The model under review builds one solid part; all positions refer to its coordinate system, in mm. Give positions to 0.01 mm unless a question says otherwise; leave off trailing zeros. Loops run counter-clockwise (first coordinate to the right, second up) from the corner with the lowest first, then second, coordinate; pieces in that order, holes last. Notation, with made-up numbers: (-11.5, 35) - (11.5, 35) arc R25 ccw to (11.5, 62) - close; hole circle Ø10 at (-10.5, -37). An arc over 180 degrees is marked (long way). Answer as a JSON object with one key per item and string values.
Autodesk Inventor part; units mm, degrees
ref_plane "YZ Plane" through (0, 0, 0) normal (1, 0, 0) x (0, 1, 0)
ref_plane "XZ Plane" through (0, 0, 0) normal (0, 1, 0) x (-1, 0, 0)
ref_plane "XY Plane" through (0, 0, 0) normal (0, 0, 1) x (1, 0, 0)
sketch "Sketch1" plane through (0, 0, 0) normal (0, 0, 1) x (1, 0, 0)
  line L0 (38.8522, 283.8417) -> (93.8522, 283.8417)
  line L1 (38.8522, 319.8417) -> (93.8522, 319.8417)
  arc A0 (10.8096, 312.4813) -> (10.8096, 291.2021) centre (13.6022, 301.8417) ccw
  line L2 (38.8522, 319.8417) -> (10.8096, 312.4813)
  line L3 (38.8522, 283.8417) -> (10.8096, 291.2021)
  arc A1 (121.8948, 291.2021) -> (121.8948, 312.4813) centre (119.1022, 301.8417) ccw
  line L4 (93.8522, 319.8417) -> (121.8948, 312.4813)
  line L5 (93.8522, 283.8417) -> (121.8948, 291.2021)
  circle A2 centre (13.6022, 301.8417) radius 5
  circle A3 centre (119.1022, 301.8417) radius 5
  circle A4 centre (58.3522, 316.3417) radius 1.5
  circle A5 centre (74.3522, 316.3417) radius 1.5
  circle A6 centre (58.3522, 287.3417) radius 1.5
  circle A7 centre (74.3522, 287.3417) radius 1.5
  dimension "d5" = 36
  dimension "d6" = 105.5
  dimension "d7" = 105.5
  dimension "d8" = 25.25
  dimension "d9" = 25.25
  dimension "d10" = 25.25
  dimension "d11" = 16
  dimension "d12" = 16
  dimension "d13" = 19.5
  dimension "d14" = 19.5
extrude "Extrusion1" add sketch "Sketch1" along normal blind 2.5
sketch "Sketch2" plane through (0, 0, 2.5) normal (0, 0, 1) x (1, 0, 0)
  circle A0 centre (13.6022, 301.8417) radius 5
  circle A1 centre (22.1022, 301.8417) radius 1
  point P0 (0, 0)
  dimension "d15" = 2
  dimension "d16" = 8.5
extrude "Extrusion2" cut sketch "Sketch2" against normal through all contours A1
pattern_circular "Circular Pattern1" count 8 over 360 about axis through (13.6022, 301.8417, 0) along (0, 0, 1) of "Extrusion2"
sketch "Sketch3" plane through (0, 0, 2.5) normal (0, 0, 1) x (1, 0, 0)
  circle A0 centre (5.1022, 301.8417) radius 1
  line L0 (93.8522, 319.8417) -> (38.8522, 319.8417)
  line L1 (66.3522, 319.8417) -> (66.3522, 283.8417)
  line L2 (38.8522, 283.8417) -> (93.8522, 283.8417)
  circle A1 centre (127.6022, 301.8417) radius 1
  point P0 (0, 0)
extrude "Extrusion3" cut sketch "Sketch3" against normal through all contours A1
pattern_circular "Circular Pattern2" count 8 over 360 about axis through (119.1022, 301.8417, 0) along (0, 0, 1) of "Extrusion3"
properties part number "Thigh" material "Aluminum-6061"
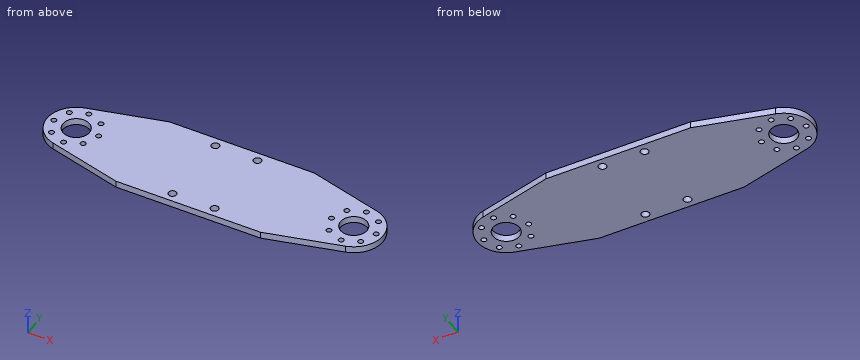
Q1. Consider section A-A, the plane y = 305.5. State the section outline as (x, z) points, plus the area to 3 significant figures.
Results:
{"outline": "(3.23, 0) - (10.19, 0) - (10.19, 2.5) - (3.23, 2.5) - close; (17.01, 0) - (115.69, 0) - (115.69, 2.5) - (17.01, 2.5) - close; (122.51, 0) - (129.48, 0) - (129.48, 2.5) - (122.51, 2.5) - close", "area": "282 mm^2"}
Q2. Consider section C-C, the plane y = 290. State the section outline as (x, z) points.
Results:
{"outline": "(15.39, 0) - (117.31, 0) - (117.31, 2.5) - (15.39, 2.5) - close"}
Q3. To check wall thickness, follow probe 1 along X at (y, z) = (303, 2.1); probe 2 along Y at (x, z) = (57.5, 2.25); probe 3 along X at (y, z) = (300, 1.1). State the ranges of each line that lie inside material, in increasing order. Write a range as [from, to].
Results:
{"probe 1": "x = [2.66, 8.74], [18.47, 114.24], [123.97, 130.04]", "probe 2": "y = [283.84, 286.11], [288.58, 315.11], [317.58, 319.84]", "probe 3": "x = [2.76, 8.95], [18.25, 114.45], [123.75, 129.95]"}
Q4. Consider section B-B, the plane z = 0.9. State how many separate pieces and enclosed holes the cut face has, plus the area to 3 significant figures.
Results:
{"separate pieces": "1", "enclosed holes": "22", "area": "3,610 mm^2"}
Q5. Clearance check with flat-ended pins moving along their axes: pin 1 Ø1.2 at (x, y) = (22.1, 301.84) entering from +Z; pin 2 Ø1.5 at (y, z) = (294.5, 1) entering from +X. State where each tip first meets the part, or that it passes through.
Results:
{"pin 1": "passes through", "pin 2": "stops at x = 127.91"}
